Geometry check sheet. Reference: drawing and pictorial views, mm from the part's lowest x, y, z. A direction names the side the tool comes from. Round coordinates to 2 decimals unless told otherwise and drop trailing zeros. Write each loop counter-clockwise with the first axis right and the second up, starting at its lowest first coordinate (ties: lowest second). Pieces come first, ordered by that corner, then holes. Notation, with made-up numbers: M 57,66.5 L 81,66.5 A19 cw 81,97.5 Z; hole C 6,-21.75 d5. An arc over 180 degrees is marked long. Answer in a Markdown table with one row per item. Add a question column.
1. Go/stop test with flat-tipped pins: pin 1 Ø6 at (x, z) = (14.5, 10.5) entering from -Y; pin 2 Ø5 at (y, z) = (24.5, 7.5) entering from +X; pin 3 Ø3 at (x, y) = (26.5, 7.5) entering from +Z. Record where each tip stops, or that it passes through.
2. Material ranges on probe 1 along Y at (x, z) = (28.5, 8.75); probe 2 along X at (y, z) = (26, 6.5); probe 3 along X at (y, z) = (25.5, 7), recorded low to high.
3. Set-up check for the marked faces 4 and 5: record each of +Z, -Z, +X, -X, +Y, -Y from which the full face is reachable in a straight line by a thin tool's end or side.
4. Draft check along X on the marked faces 1, 2 and 3. Enter one of: pulls with the +X half, pulls with the -X half, needs draft (parallel to the pull), parting line crosses it, or undercut.
5. Sectioned sample at B-B on x = 18.5. Record the cut outline in (y, z).
6. Sectioned sample at A-A on y = 28.5. Record the cut outline in (x, z).
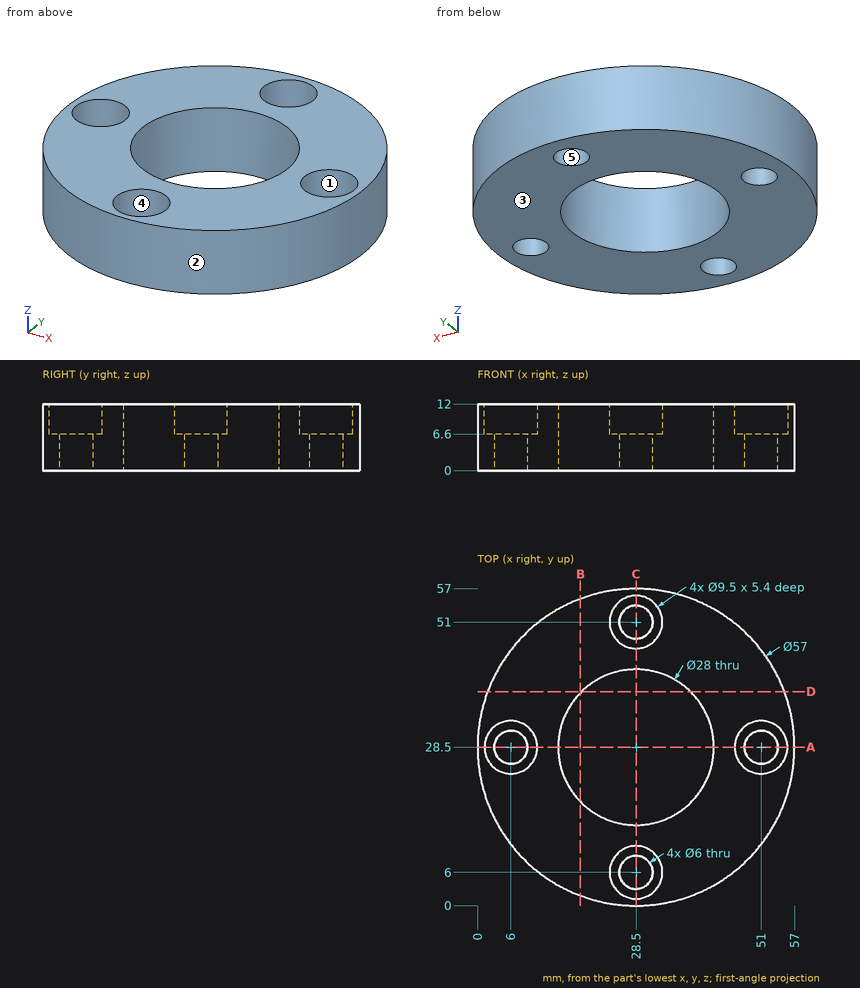
Geometry check:
| question | item | result |
|---|---|---|
| 1 | pin 1 | stops at y = 2.21 |
| 1 | pin 2 | stops at x = 56.96 |
| 1 | pin 3 | stops at z = 6.6 |
| 2 | probe 1 | y = 0 to 1.25, 10.75 to 14.5, 42.5 to 46.25, 55.75 to 57 |
| 2 | probe 2 | x = 0.11 to 4.34, 7.66 to 14.73, 42.27 to 49.34, 52.66 to 56.89 |
| 2 | probe 3 | x = 0.16 to 2.32, 9.68 to 14.83, 42.17 to 47.32, 54.68 to 56.84 |
| 3 | face 4 | +Z |
| 3 | face 5 | +Z, -Z |
| 4 | face 1 | undercut |
| 4 | face 2 | parting line crosses it |
| 4 | face 3 | needs draft |
| 5 | outline | M 1.81,0 L 18.7,0 L 18.7,12 L 1.81,12 Z; M 38.3,0 L 55.19,0 L 55.19,12 L 38.3,12 Z |
| 6 | outline | M 0,0 L 3,0 L 3,6.6 L 1.25,6.6 L 1.25,12 L 0,12 Z; M 9,0 L 14.5,0 L 14.5,12 L 10.75,12 L 10.75,6.6 L 9,6.6 Z; M 42.5,0 L 48,0 L 48,6.6 L 46.25,6.6 L 46.25,12 L 42.5,12 Z; M 54,0 L 57,0 L 57,12 L 55.75,12 L 55.75,6.6 L 54,6.6 Z |
